Input: part model. Units: mm. Frame: model coordinates. Face numbers are marked on the shaded views. A direction names the side the tool comes from. Coordinates: 2 decimals unless noted, no trailing zeros. Order: outer loops, then holes, each group sorted by start corner. A loop starts at its lowest first (then second) coordinate and runs counter-clockwise, first axis right, second up.
from build123d import *

# Parameters (mm, degrees)
SKETCH1_R               = 2.5
BOSS_EXTRUDE1_DEPTH     = 35
SKETCH2_R               = 1.5
CUT_EXTRUDE1_DEPTH      = 3.5
CUT_EXTRUDE1_DEPTH_BACK = 3.5
SKETCH4_R               = 1.5
BOSS_EXTRUDE3_DEPTH     = 15


with BuildPart() as part:
    # Sketch1 → Boss-Extrude1 (new body)
    with BuildSketch(Plane(origin=(0, 0, 0), x_dir=(1, 0, 0), z_dir=(0, 1, 0))):
        Circle(SKETCH1_R)
    extrude(amount=BOSS_EXTRUDE1_DEPTH)

    # Sketch2 → Cut-Extrude1 (cut, two sides)
    with BuildSketch(Plane(origin=(0, 0, 0), x_dir=(0, 0, -1), z_dir=(1, 0, 0))) as cut_extrude1_sk:
        with Locations((0, 5)):
            Circle(SKETCH2_R)
    extrude(amount=CUT_EXTRUDE1_DEPTH, mode=Mode.SUBTRACT)
    extrude(cut_extrude1_sk.sketch, amount=-CUT_EXTRUDE1_DEPTH_BACK, mode=Mode.SUBTRACT)

    # Sketch4 → Boss-Extrude3 (add)
    with BuildSketch(Plane.XY):
        with Locations((0, 30)):
            Circle(SKETCH4_R)
    extrude(amount=BOSS_EXTRUDE3_DEPTH)


solid = part.part
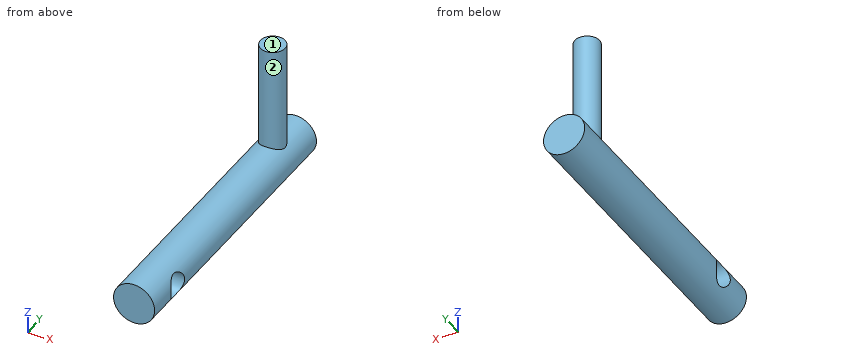
Item 1: Access query for the marked faces 1 and 2. Directions: +Z, -Z, +X, -X, +Y, -Y. A direction counts if a zero-diameter tool reaches every point of the face in a straight line with its end or side. Return the directions, or none.
Response values:
face 1: +Z, +X, -X, +Y, -Y
face 2: +Z
Item 2: Cut plane C-C on y = 5. Return loops of the section in (x, z).
Response values:
outline: (-2, -1.5) arc R2.5 ccw to (2, -1.5) - close; (-2, 1.5) - (2, 1.5) arc R2.5 ccw to start
Item 3: Pin query (flat end, axial travel): pin 1 Ø2 at (y, z) = (30, 1.5) entering from -X; pin 2 Ø1.5 at (x, y) = (-1, 16) entering from -Z; pin 3 Ø1 at (y, z) = (26.5, 2.5) entering from +X. Return the tip coordinate at first contact, or that it passes through.
Response values:
pin 1: stops at x = -2.45
pin 2: stops at z = -2.49
pin 3: stops at x = 1.5
Item 4: Cut plane A-A on z = 0. Return loops of the section in (x, y), then the cut area to 3 significant figures.
Response values:
outline: (-2.5, 0) - (2.5, 0) - (2.5, 3.5) - (-2.5, 3.5) - close; (-2.5, 6.5) - (2.5, 6.5) - (2.5, 35) - (-2.5, 35) - close
area: 160 mm2
Item 5: Cut plane D-D on x = -0.75. Return loops of the section in (y, z), then the cut area to 3 significant figures.
Response values:
outline: (0, -2.38) - (35, -2.38) - (35, 2.38) - (31.3, 2.38) - (31.3, 15) - (28.7, 15) - (28.7, 2.38) - (0, 2.38) - close; hole circle Ø3 at (5, 0)
area: 193 mm2
Item 6: Cut plane B-B on x = 1. Return loops of the section in (y, z).
Response values:
outline: (0, -2.29) - (35, -2.29) - (35, 2.29) - (31.12, 2.29) - (31.12, 15) - (28.88, 15) - (28.88, 2.29) - (0, 2.29) - close; hole circle Ø3 at (5, 0)
Item 7: Ray query, probe 1 along Y at (x, z) = (-1.35, 0); probe 2 along Z at (x, y) = (-0.9, 5); probe 3 along Y at (x, z) = (0, 10.5). Return the intervals inside material, ascending.
Response values:
probe 1: y = 0 to 3.5, 6.5 to 35
probe 2: z = -2.33 to -1.5, 1.5 to 2.33
probe 3: y = 28.5 to 31.5
